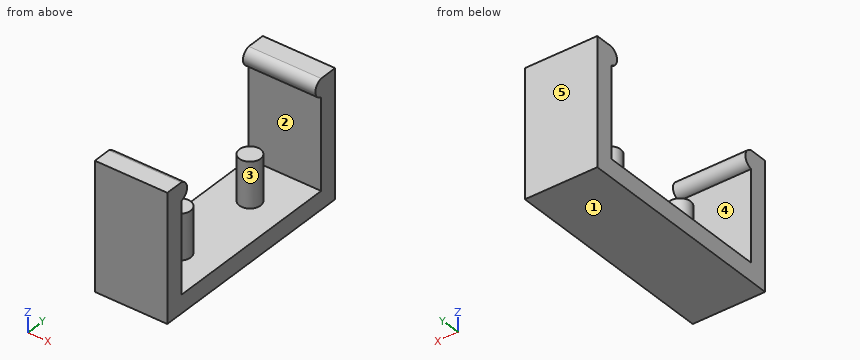
from build123d import *

# Parameters (mm, degrees)
SKETCH1_W           = 8
SKETCH1_H           = 24
BOSS_EXTRUDE1_DEPTH = 2
SKETCH2_W           = 8
SKETCH2_H           = 2
BOSS_EXTRUDE2_DEPTH = 12
BOSS_EXTRUDE4_DEPTH = 8
SKETCH4_R           = 1.175
BOSS_EXTRUDE5_DEPTH = 5


with BuildPart() as part:
    # Sketch1 → Boss-Extrude1 (new body)
    with BuildSketch(Plane.XY):
        Rectangle(SKETCH1_W, SKETCH1_H)
    extrude(amount=BOSS_EXTRUDE1_DEPTH)

    # Sketch2 → Boss-Extrude2 (add)
    with BuildSketch(Plane.XY.offset(2)):
        with Locations((0, 11)):
            Rectangle(SKETCH2_W, SKETCH2_H)
        with Locations((0, -11)):
            Rectangle(SKETCH2_W, SKETCH2_H)
    extrude(amount=BOSS_EXTRUDE2_DEPTH)

    # Sketch3 → Boss-Extrude4 (add)
    with BuildSketch(Plane(origin=(4, 0, 0), x_dir=(0, 0, -1), z_dir=(1, 0, 0))):
        with BuildLine():
            ThreePointArc((-12, -10), (-13, -9.180997512), (-14, -10))
            Line((-14, -10), (-12, -10))
        make_face()
        with BuildLine():
            ThreePointArc((-12, 10), (-13, 9.180997512), (-14, 10))
            Line((-14, 10), (-12, 10))
        make_face()
    extrude(amount=-BOSS_EXTRUDE4_DEPTH)

    # Sketch4 → Boss-Extrude5 (add)
    with BuildSketch(Plane.XY.offset(2)):
        with Locations((0, -5)):
            Circle(SKETCH4_R)
        with Locations((0, 5)):
            Circle(SKETCH4_R)
    extrude(amount=BOSS_EXTRUDE5_DEPTH)


solid = part.part
Design review of the part built by this model. Coordinates are the model's own, in mm. Face numbers are marked on the shaded views. A direction names the side the tool comes from. Coordinates: 2 decimals unless noted, no trailing zeros. Loops run counter-clockwise (first coordinate to the right, second up) from the corner with the lowest first, then second, coordinate; pieces in that order, holes last.
Item 1: Draft analysis for pull direction Z (two halves, no side actions). For the marked faces 1, 2 and 3, state which applies: pulls with the +Z half, pulls with the -Z half, needs draft (parallel to the pull), parting line crosses it, or undercut.
Completed:
face 1: pulls with the -Z half
face 2: undercut
face 3: needs draft
Item 2: For the marked faces 4 and 5, list the 3-axis set-ups (+Z, -Z, +X, -X, +Y, -Y) from which the entire face can be reached by the end or side of a thin tool; tool diameter is ignored.
Completed:
face 4: +X, -X
face 5: +Z, -Z, +X, -X, +Y
Item 3: Add section A-A (y = 5). Write out the cut boundary in (x, z) (3 decimals).
Completed:
outline: (-4, 0) - (4, 0) - (4, 2) - (1.175, 2) - (1.175, 7) - (-1.175, 7) - (-1.175, 2) - (-4, 2) - close
Item 4: Add section C-C (x = -3). Write out the cut boundary in (y, z).
Completed:
outline: (-12, 0) - (12, 0) - (12, 14) - (10, 14) arc R1.02 ccw to (10, 12) - (10, 2) - (-10, 2) - (-10, 12) arc R1.02 ccw to (-10, 14) - (-12, 14) - close
Item 5: Clearance check with flat-ended pins moving along their axes: pin 1 (1.5 mm diameter, centred on x = -1.5, y = -1, fed in from +Z); pin 2 (2.5 mm diameter, centred on x = 0, y = 5, fed in from +Z). State where each tip first meets the part, or that it passes through.
Completed:
pin 1: stops at z = 2
pin 2: stops at z = 7
Item 6: Add section D-D (z = 12.5). Write out the cut boundary in (x, y), and give its area (3 significant figures).
Completed:
outline: (-4, -12) - (4, -12) - (4, -9.31) - (-4, -9.31) - close; (-4, 9.31) - (4, 9.31) - (4, 12) - (-4, 12) - close
area: 43.0 mm2
Item 7: Add section B-B (z = 4.5). Write out the cut boundary in (x, y) (3 decimals), and give its area (3 significant figures).
Completed:
outline: (-4, -12) - (4, -12) - (4, -10) - (-4, -10) - close; (-4, 10) - (4, 10) - (4, 12) - (-4, 12) - close; circle Ø2.35 at (0, -5); circle Ø2.35 at (0, 5)
area: 40.7 mm2
Item 8: Wall thickness on L1, parallel to Y at x = -2, z = 10.75; L2, parallel to Y at x = -0.5, z = 4.75; L3, parallel to Z at x = -3.5, y = 8: over which ranges is each line inside the solid? List them lowest first.
Completed:
L1: y = -12 to -10, 10 to 12
L2: y = -12 to -10, -6.06 to -3.94, 3.94 to 6.06, 10 to 12
L3: z = 0 to 2
